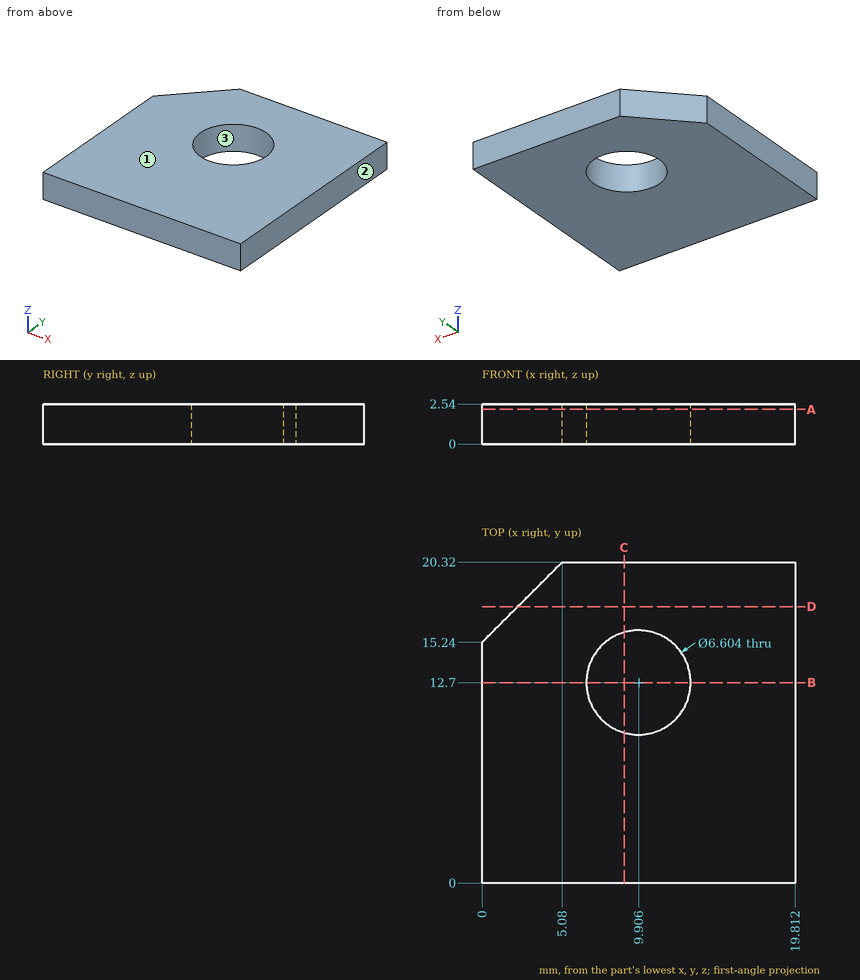
Drawing for the job (mm, zero at the part's lowest x, y, z). Coordinates: 2 decimals unless noted, no trailing zeros. Order: outer loops, then holes, each group sorted by start corner. A loop starts at its lowest first (then second) coordinate and runs counter-clockwise, first axis right, second up.
Item 1: Band-saw the part on D-D on y = 17.5. List the corners of the cut face in (x, z), plus the area to 3 significant figures.
Check sheet entries:
outline: (2.26, 0) - (19.81, 0) - (19.81, 2.54) - (2.26, 2.54) - close
area: 44.6 mm2
Item 2: Two-plate mould, pull along X, no slides. Class the marked faces 1, 2 and 3: +X half, -X half, draft (parallel to the pull), parting line (faces both ways), or undercut.
Check sheet entries:
face 1: draft
face 2: +X half
face 3: undercut
Item 3: Band-saw the part on C-C on x = 9. List the corners of the cut face in (y, z), plus the area to 3 significant figures.
Check sheet entries:
outline: (0, 0) - (9.52, 0) - (9.52, 2.54) - (0, 2.54) - close; (15.88, 0) - (20.32, 0) - (20.32, 2.54) - (15.88, 2.54) - close
area: 35.5 mm2
Item 4: Band-saw the part on B-B on y = 12.7. List the corners of the cut face in (x, z), plus the area to 3 significant figures.
Check sheet entries:
outline: (0, 0) - (6.6, 0) - (6.6, 2.54) - (0, 2.54) - close; (13.21, 0) - (19.81, 0) - (19.81, 2.54) - (13.21, 2.54) - close
area: 33.5 mm2
Item 5: Pin check, flat tip, straight feed: pin 1 Ø10.5 at (x, y) = (9.906, 12.7) entering from +Z. Stop position of the tip, or through.
Check sheet entries:
pin 1: stops at z = 2.54
Item 6: Drill centre lines: L1, parallel to X at y = 10, z = 0.4; L2, parallel to Y at x = 8.25, z = 1.9; L3, parallel to Y at x = 11, z = 0.8. Where is each one in solid material? Low to high.
Check sheet entries:
L1: x = 0 to 8.01, 11.81 to 19.81
L2: y = 0 to 9.84, 15.56 to 20.32
L3: y = 0 to 9.58, 15.82 to 20.32
Item 7: Band-saw the part on A-A on z = 2.2. List the corners of the cut face in (x, y), plus the area to 3 significant figures.
Check sheet entries:
outline: (0, 0) - (19.81, 0) - (19.81, 20.32) - (5.08, 20.32) - (0, 15.24) - close; hole circle Ø6.6 at (9.91, 12.7)
area: 355 mm2
